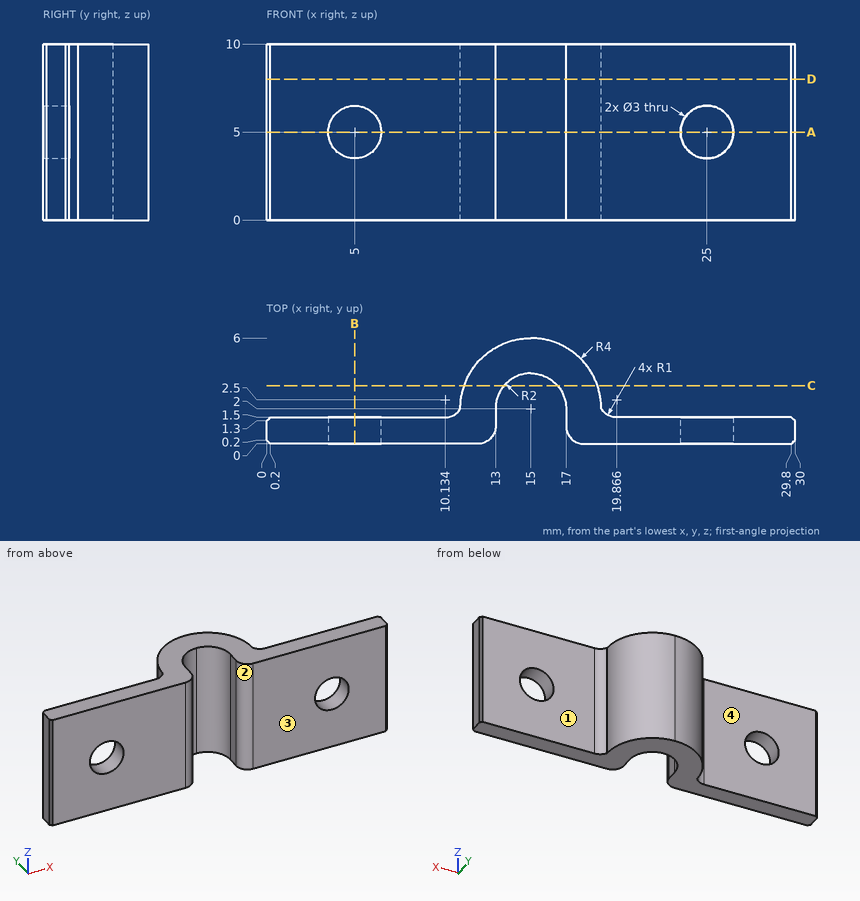
The drawing under review shows one solid part. Ordinate dimensions are in mm from its lowest x, y, z. A direction names the side the tool comes from. Round coordinates to 2 decimals unless told otherwise and drop trailing zeros. Loops run counter-clockwise (first coordinate to the right, second up) from the corner with the lowest first, then second, coordinate; pieces in that order, holes last. Notation, with made-up numbers: M 19,-7 L 61,-7 A8 ccw 61,8 Z; hole C 3,-39 d11. An arc over 180 degrees is marked long. Answer as CSV lines item,"result". Start each with the question number.
Item 1: Insertion check: P1, Ø1, axis at y = 5, z = 6, coming from the +X side; P2, Ø5, axis at x = 27.5, z = 3.5, coming from the +Y side; P3, Ø2, axis at x = 13.5, z = 4, coming from the -Y side; P4, Ø1.1, axis at y = 1.5, z = 3, coming from the -X side. Each pin has a flat end and moves straight along its axis. Give the tip position at first contact, or say it passes through.
Item 2: For the marked faces 3 and 4, list the 3-axis set-ups (+Z, -Z, +X, -X, +Y, -Y) from which the entire face can be reached by the end or side of a thin tool; tool diameter is ignored.
Item 3: Wall thickness on line 1 (Z direction, x = 5, y = 1.1); line 2 (X direction, y = 2.1, z = 5.75); line 3 (Y direction, x = 20.75, z = 5.75): over which ranges is each line inside the solid? List them lowest first. Write a range as [from, to].
Item 4: Mouldability with a two-part tool opening along X and no side actions: class the marked faces 1 and 2 as released by +X, released by -X, zero draft, split by the parting line, or undercut.
Item 5: Consider section C-C (y = 3.3). Write out the cut boundary in (x, z), then the cut area to 3 significant figures.
Item 6: Consider section D-D (z = 8). Write out the cut boundary in (x, y).
Item 7: Consider section B-B (x = 5). Write out the cut boundary in (y, z).
Item 8: Consider section A-A (z = 5). Write out the cut boundary in (x, y), then the cut area to 3 significant figures.
Answer:
1,P1,"stops at x = 18.12"
1,P2,"stops at y = 1.5"
1,P3,"stops at y = 0.13"
1,P4,"stops at x = 0"
2,face 3,"+Z, -Z, +X, -X, -Y"
2,face 4,"+Z, -Z, -X, +Y"
3,line 1,"z = [0, 3.5], [6.5, 10]"
3,line 2,"x = [11, 13], [17, 19]"
3,line 3,"y = [0, 1.5]"
4,face 1,"zero draft"
4,face 2,"undercut"
5,outline,"M 11.22,0 L 13.48,0 L 13.48,10 L 11.22,10 Z; M 16.52,0 L 18.78,0 L 18.78,10 L 16.52,10 Z"
5,area,"45.3 mm^2"
6,outline,"M 0,0.2 L 0.2,0 L 12,0 A1 ccw 13,1 L 13,2 A2 cw 17,2 L 17,1 A1 ccw 18,0 L 29.8,0 L 30,0.2 L 30,1.3 L 29.8,1.5 L 19.87,1.5 A1 cw 19,2 A4 ccw 11,2 A1 cw 10.13,1.5 L 0.2,1.5 L 0,1.3 Z"
7,outline,"M 0,0 L 1.5,0 L 1.5,3.5 L 0,3.5 Z; M 0,6.5 L 1.5,6.5 L 1.5,10 L 0,10 Z"
8,outline,"M 0,0.2 L 0.2,0 L 3.5,0 L 3.5,1.5 L 0.2,1.5 L 0,1.3 Z; M 6.5,0 L 12,0 A1 ccw 13,1 L 13,2 A2 cw 17,2 L 17,1 A1 ccw 18,0 L 23.5,0 L 23.5,1.5 L 19.87,1.5 A1 cw 19,2 A4 ccw 11,2 A1 cw 10.13,1.5 L 6.5,1.5 Z; M 26.5,0 L 29.8,0 L 30,0.2 L 30,1.3 L 29.8,1.5 L 26.5,1.5 Z"
8,area,"50.6 mm^2"
